```python
from build123d import *

# Parameters (mm, degrees)
BOSS_EXTRUDE1_DEPTH     = 11.5
CUT_EXTRUDE5_START      = -32.140020188
SKETCH7_R               = 4.3
CUT_EXTRUDE5_DEPTH      = 40.640020188
CUT_EXTRUDE6_START      = -3.8
SKETCH7_3_R             = 7
SKETCH7_3_R_2           = 4.3
CUT_EXTRUDE6_DEPTH      = 28.340020336
SKETCH8_R               = 1.65
CUT_EXTRUDE7_DEPTH      = 12.5000001
CUT_EXTRUDE7_DEPTH_BACK = 12.5000001
CUT_EXTRUDE8_START      = -5
SKETCH8_3_R             = 1.65
CUT_EXTRUDE8_DEPTH      = 7.5000001
CUT_EXTRUDE9_START      = 5
SKETCH8_4_R             = 1.65
CUT_EXTRUDE9_DEPTH      = 7.5000001


with BuildPart() as part:
    # Sketch4 → Boss-Extrude1 (new body, symmetric)
    with BuildSketch(Plane.XY):
        with BuildLine():
            ThreePointArc((-18.879751058, 25.243712088), (0, 31.522848856), (18.879751058, 25.243712088))
            Line((18.879751058, 25.243712088), (8.27314934, 14.637110371))
            Line((8.27314934, 14.637110371), (-8.27314934, 14.637110371))
            Line((-8.27314934, 14.637110371), (-18.879751058, 25.243712088))
        make_face()
    extrude(amount=BOSS_EXTRUDE1_DEPTH, both=True)

    # Sketch4_3 → Revolve1 (revolve)
    with BuildSketch(Plane.XY):
        Polygon((-16.617009358, 22.980970389), (-17.465537495, 23.829498526), (-18.172644276, 23.122391745), (-17.324116139, 22.273863607), align=None)
    revolve1 = revolve(axis=Axis((-14.28355698, 19.233304448, 0), (0.707106781, 0.707106781, 0)))

    # Sketch7 → Cut-Extrude5 (cut)
    with BuildSketch(Plane(origin=(3.181980515, 3.181980515, 0), x_dir=(0, 0, 1), z_dir=(-0.707106781, -0.707106781, 0)).offset(CUT_EXTRUDE5_START)):
        with Locations((0, 23.7)):
            Circle(SKETCH7_R)
    cut_extrude5 = extrude(amount=CUT_EXTRUDE5_DEPTH, mode=Mode.SUBTRACT)

    # Sketch7_3 → Cut-Extrude6 (cut, through all)
    with BuildSketch(Plane(origin=(3.181980515, 3.181980515, 0), x_dir=(0, 0, 1), z_dir=(-0.707106781, -0.707106781, 0)).offset(CUT_EXTRUDE6_START)):
        with Locations((0, 23.7)):
            Circle(SKETCH7_3_R)
        with Locations((0, 23.7)):
            Circle(SKETCH7_3_R_2, mode=Mode.SUBTRACT)
    cut_extrude6 = extrude(amount=-CUT_EXTRUDE6_DEPTH, mode=Mode.SUBTRACT)

    # Mirror2: Revolve1, Cut-Extrude5, Cut-Extrude6 across plane
    add(revolve1.mirror(Plane(origin=(0, 0, 0), x_dir=(0, 0, 1), z_dir=(1, 0, 0))))
    add(cut_extrude5.mirror(Plane(origin=(0, 0, 0), x_dir=(0, 0, 1), z_dir=(1, 0, 0))), mode=Mode.SUBTRACT)
    add(cut_extrude6.mirror(Plane(origin=(0, 0, 0), x_dir=(0, 0, 1), z_dir=(1, 0, 0))), mode=Mode.SUBTRACT)

    # Sketch8 → Cut-Extrude7 (cut, two sides)
    with BuildSketch(Plane.XY) as cut_extrude7_sk:
        with Locations((-3, 18)):
            Circle(SKETCH8_R)
        with Locations((3, 18)):
            Circle(SKETCH8_R)
    extrude(amount=CUT_EXTRUDE7_DEPTH, mode=Mode.SUBTRACT)
    extrude(cut_extrude7_sk.sketch, amount=-CUT_EXTRUDE7_DEPTH_BACK, mode=Mode.SUBTRACT)

    # Sketch8_3 → Cut-Extrude8 (cut, through all)
    with BuildSketch(Plane.XY.offset(CUT_EXTRUDE8_START)):
        Polygon((-6.883130466, 18), (-4.941565233, 14.637110371), (-1.058434767, 14.637110371), (0.883130466, 18), (-1.058434767, 21.362889629), (-4.941565233, 21.362889629), align=None)
        with Locations((-3, 18)):
            Circle(SKETCH8_3_R, mode=Mode.SUBTRACT)
    extrude(amount=-CUT_EXTRUDE8_DEPTH, mode=Mode.SUBTRACT)

    # Sketch8_4 → Cut-Extrude9 (cut, through all)
    with BuildSketch(Plane.XY.offset(CUT_EXTRUDE9_START)):
        Polygon((6.883130466, 18), (4.941565233, 21.362889629), (1.058434767, 21.362889629), (-0.883130466, 18), (1.058434767, 14.637110371), (4.941565233, 14.637110371), align=None)
        with Locations((3, 18)):
            Circle(SKETCH8_4_R, mode=Mode.SUBTRACT)
    extrude(amount=CUT_EXTRUDE9_DEPTH, mode=Mode.SUBTRACT)


solid = part.part
```
Here's how the part is built. I have some questions about the finished solid (model axes, mm). A direction names the side the tool comes from. Coordinates: 2 decimals unless noted, no trailing zeros. Order: outer loops, then holes, each group sorted by start corner. A loop starts at its lowest first (then second) coordinate and runs counter-clockwise, first axis right, second up.
Item 1: Thinking about a two-plate mould opening in X: for faces 6 (the face through (14.27, 19.22, -4.46)), 7 (the face through (3, 21.363, 8)), 8 (the face through (-0.28, 31.52, -7.51)), which applies, pulls with the +X half, pulls with the -X half, needs draft (parallel to the pull), parting line crosses it, or undercut?
Response values:
face 6: pulls with the +X half
face 7: undercut
face 8: parting line crosses it
Item 2: Which directions (+Z, -Z, +X, -X, +Y, -Y) give clear straight access to the entire face, cutting with the end or side of a thin tool? Please do faces 1 (the face through (0, 23, 11.5)), 2 (the face through (-0.1, 19.7, -8.2)), 3 (the face through (-14.27, 19.22, -4.46)), 4 (the face through (-8.7, 20.44, -3.21)), 5 (the face through (5, 18, 5)).
Response values:
face 1: +Z, +X, -X, +Y, -Y
face 2: -Z
face 3: +Z, -Z, -X, -Y
face 4: none
face 5: +Z
Item 3: I need wall thicknesses on probe 1 along X at (y, z) = (18, 8.25); probe 2 along Z at (x, y) = (8, 26); probe 3 along X at (y, z) = (25.5, 3). Which ranges of each line are inside material? Lowest first, please.
Response values:
probe 1: x = -11.64 to -4.65, -1.35 to -0.88, 6.88 to 11.64
probe 2: z = -11.5 to -6.99, 6.99 to 11.5
probe 3: x = -18.53 to -13.76, 13.76 to 18.53
Item 4: If we section it at A-A, the plane z = -2.75: Give the number of separate pieces and of enclosed holes in the cut face, then the cut area to 3 significant figures.
Response values:
separate pieces: 3
enclosed holes: 2
area: 136 mm2
Item 5: If we section it at B-B, the plane z = 9: List the corners of the cut face in (x, y) for me, then the cut area to 3 significant figures.
Response values:
outline: (-18.88, 25.24) - (-8.27, 14.64) - (1.06, 14.64) - (-0.88, 18) - (1.06, 21.36) - (4.94, 21.36) - (6.88, 18) - (4.94, 14.64) - (8.27, 14.64) - (18.88, 25.24) arc R31.52 ccw to start; hole circle Ø3.3 at (-3, 18)
area: 402 mm2
Item 6: I'm going to push flat-ended pins straight in: pin 1 Ø3.5 at (x, y) = (1.5, 19.5) entering from +Z; pin 2 Ø1.9 at (x, z) = (-3.5, -8.5) entering from -Y; pin 3 Ø6 at (y, z) = (29, 3) entering from +X; pin 4 Ø2 at (x, z) = (-12.5, -6.5) entering from +Y. Where does each tip first touch, or does it pass through?
Response values:
pin 1: stops at z = 11.5
pin 2: stops at y = 21.36
pin 3: stops at x = 17.82
pin 4: stops at y = 29.35
